from build123d import *

# Parameters (mm, degrees)
SKETCH1_R           = 10.4
BOSS_EXTRUDE1_DEPTH = 2.25
SKETCH2_R           = 4.4
BOSS_EXTRUDE2_DEPTH = 3.3
SKETCH3_R           = 1.5
SKETCH3_R_2         = 0.875
CUT_EXTRUDE1_DEPTH  = 5.55
SKETCH4_R           = 2.925
CUT_EXTRUDE2_DEPTH  = 1.7
SKETCH5_R           = 2.95
CUT_EXTRUDE3_DEPTH  = 3


with BuildPart() as part:
    # Sketch1 → Boss-Extrude1 (new body)
    with BuildSketch(Plane.XY):
        with Locations((9.62, 10)):
            Circle(SKETCH1_R)
    extrude(amount=BOSS_EXTRUDE1_DEPTH)

    # Sketch2 → Boss-Extrude2 (add)
    with BuildSketch(Plane(origin=(0, 0, 0), x_dir=(-1, 0, 0), z_dir=(0, 0, -1))):
        with Locations((-9.62, 10)):
            Circle(SKETCH2_R)
    extrude(amount=BOSS_EXTRUDE2_DEPTH)

    # Sketch3 → Cut-Extrude1 (cut)
    with BuildSketch(Plane.XY.offset(2.25)):
        with Locations((9.62, 10)):
            Circle(SKETCH3_R)
        with Locations((9.62, 2.715)):
            Circle(SKETCH3_R_2)
        with Locations((5.97, 2.715)):
            Circle(SKETCH3_R_2)
        with Locations((13.27, 2.715)):
            Circle(SKETCH3_R_2)
        with Locations((2.335, 6.35)):
            Circle(SKETCH3_R_2)
        with Locations((2.335, 10)):
            Circle(SKETCH3_R_2)
        with Locations((2.335, 13.65)):
            Circle(SKETCH3_R_2)
        with Locations((5.97, 17.285)):
            Circle(SKETCH3_R_2)
        with Locations((9.62, 17.285)):
            Circle(SKETCH3_R_2)
        with Locations((13.27, 17.285)):
            Circle(SKETCH3_R_2)
        with Locations((16.905, 13.65)):
            Circle(SKETCH3_R_2)
        with Locations((16.905, 10)):
            Circle(SKETCH3_R_2)
        with Locations((16.905, 6.35)):
            Circle(SKETCH3_R_2)
    extrude(amount=-CUT_EXTRUDE1_DEPTH, mode=Mode.SUBTRACT)

    # Sketch4 → Cut-Extrude2 (cut)
    with BuildSketch(Plane.XY.offset(2.25)):
        with Locations((9.62, 10)):
            Circle(SKETCH4_R)
    extrude(amount=-CUT_EXTRUDE2_DEPTH, mode=Mode.SUBTRACT)

    # Sketch5 → Cut-Extrude3 (cut)
    with BuildSketch(Plane(origin=(0, 0, -3.3), x_dir=(-1, 0, 0), z_dir=(0, 0, -1))):
        with Locations((-9.62, 10)):
            Circle(SKETCH5_R)
    extrude(amount=-CUT_EXTRUDE3_DEPTH, mode=Mode.SUBTRACT)


solid = part.part
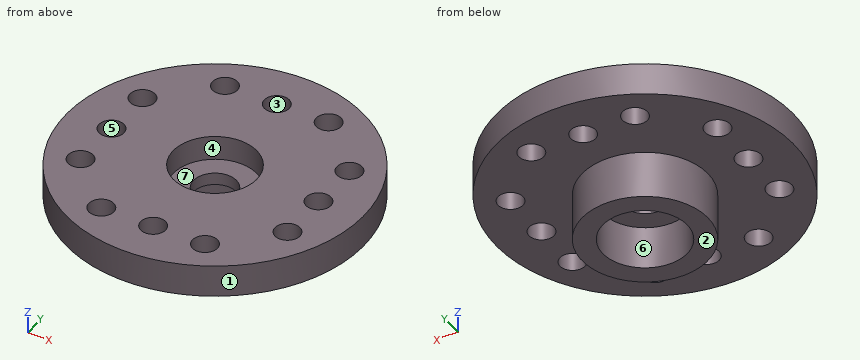
Model file for the job. Use its own axes, mm. Face numbers are marked on the shaded views. A direction names the side the tool comes from. Give positions to 0.01 mm unless a question says otherwise; leave off trailing zeros. Write each loop counter-clockwise with the first axis right and the second up, starting at its lowest first coordinate (ties: lowest second). Pieces come first, ordered by that corner, then holes. Notation, with made-up numbers: (81.25, 42) -> (100.25, 42) arc R5 ccw to (100.25, 50) -> close; hole circle Ø1 at (-0.75, 86.5). An arc over 180 degrees is marked (long way). Write item = value, one per line.
(1) Slice it at B-B, the plane x = 9.62. Give the cut face in (y, z) (3 decimals).
Determined:
outline = (-0.4, 0) -> (1.84, 0) -> (1.84, 2.25) -> (-0.4, 2.25) -> close; (3.59, 0) -> (5.6, 0) -> (5.6, -3.3) -> (7.05, -3.3) -> (7.05, -0.3) -> (8.5, -0.3) -> (8.5, 0.55) -> (7.075, 0.55) -> (7.075, 2.25) -> (3.59, 2.25) -> close; (11.5, -0.3) -> (12.95, -0.3) -> (12.95, -3.3) -> (14.4, -3.3) -> (14.4, 0) -> (16.41, 0) -> (16.41, 2.25) -> (12.925, 2.25) -> (12.925, 0.55) -> (11.5, 0.55) -> close; (18.16, 0) -> (20.4, 0) -> (20.4, 2.25) -> (18.16, 2.25) -> close
(2) Probe line 1 along Y through (x, z) = (9.62, 0.95) (3 decimals); line 2 along Y through (x, z) = (17, 0.7); line 3 along X through (y, z) = (13.25, 1.25). List the from-to ranges inside material, lowest first.
Determined:
line_1 = -0.4 to 1.84, 3.59 to 7.075, 12.925 to 16.41, 18.16 to 20.4
line_2 = 2.67 to 5.48, 7.22 to 9.13, 10.87 to 12.78, 14.52 to 17.33
line_3 = -0.26 to 1.56, 3.11 to 16.13, 17.68 to 19.5
(3) Tool access for the marked faces 5, 6 and 7: list every direction of +Z, -Z, +X, -X, +Y, -Y with a clear straight run to the whole face (end or side of a thin tool).
Determined:
face_5 = +Z, -Z
face_6 = -Z
face_7 = +Z
(4) Slice it at C-C, the plane y = 6. Give the cut face in (x, z).
Determined:
outline = (0.02, 0) -> (1.53, 0) -> (1.53, 2.25) -> (0.02, 2.25) -> close; (3.14, 0) -> (7.79, 0) -> (7.79, -3.3) -> (11.45, -3.3) -> (11.45, 0) -> (16.1, 0) -> (16.1, 2.25) -> (3.14, 2.25) -> close; (17.71, 0) -> (19.22, 0) -> (19.22, 2.25) -> (17.71, 2.25) -> close
(5) Mould opens along Y. For the marked faces 1, 2, 3 and 4 say: released by +Y, released by -Y, zero draft, split by the parting line, or undercut.
Determined:
face_1 = split by the parting line
face_2 = zero draft
face_3 = undercut
face_4 = undercut
(6) Slice it at D-D, the plane x = 5.97. Give the cut face in (y, z), then the cut area to 3 significant figures.
Determined:
outline = (0.26, 0) -> (1.84, 0) -> (1.84, 2.25) -> (0.26, 2.25) -> close; (3.59, 0) -> (7.54, 0) -> (7.54, -3.3) -> (12.46, -3.3) -> (12.46, 0) -> (16.41, 0) -> (16.41, 2.25) -> (3.59, 2.25) -> close; (18.16, 0) -> (19.74, 0) -> (19.74, 2.25) -> (18.16, 2.25) -> close
area = 52.2 mm2
(7) Flat gauge pins, fed straight in: P1, Ø2.5, axis at x = 16.905, y = 6.35, coming from the -Z side; P2, Ø2, axis at y = 15.5, z = -1.5, coming from the +X side; P3, Ø3.5, axis at x = 9.62, y = 10, coming from the +Z side; P4, Ø2, axis at x = 3.5, z = 0, coming from the +Y side. Where does each tip first touch, or does it go through?
Determined:
P1 = 0
P2 = through
P3 = 0.55
P4 = 19.05
(8) Slice it at A-A, the plane y = 10. Give the cut face in (x, z) (3 decimals).
Determined:
outline = (-0.78, 0) -> (1.46, 0) -> (1.46, 2.25) -> (-0.78, 2.25) -> close; (3.21, 0) -> (5.22, 0) -> (5.22, -3.3) -> (6.67, -3.3) -> (6.67, -0.3) -> (8.12, -0.3) -> (8.12, 0.55) -> (6.695, 0.55) -> (6.695, 2.25) -> (3.21, 2.25) -> close; (11.12, -0.3) -> (12.57, -0.3) -> (12.57, -3.3) -> (14.02, -3.3) -> (14.02, 0) -> (16.03, 0) -> (16.03, 2.25) -> (12.545, 2.25) -> (12.545, 0.55) -> (11.12, 0.55) -> close; (17.78, 0) -> (20.02, 0) -> (20.02, 2.25) -> (17.78, 2.25) -> close
